Verification items for the finished model (mm, model axes). Give positions to 0.01 mm unless a question says otherwise; leave off trailing zeros. Loops run counter-clockwise (first coordinate to the right, second up) from the corner with the lowest first, then second, coordinate; pieces in that order, holes last. Notation, with made-up numbers: M 13,-14.5 L 49,-14.5 A23 ccw 49,-6.5 Z; hole C 43,44.25 d8. An arc over 180 degrees is marked long. Answer in a Markdown table with one row per item.
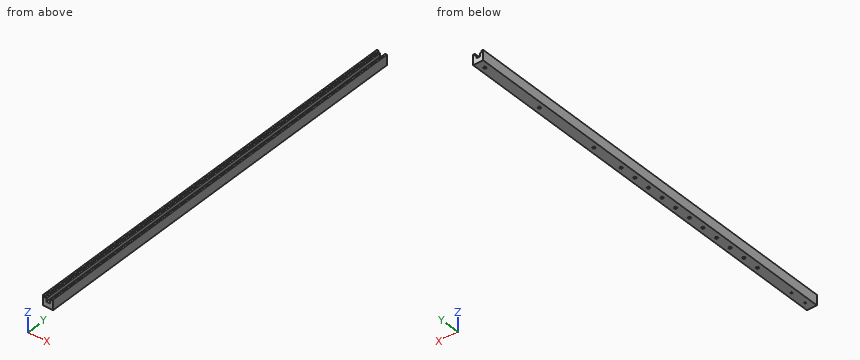
```python
from build123d import *

# Parameters (mm, degrees)
SKETCH1_W                 = 30
SKETCH1_H                 = 30
BOSS_EXTRUDE1_DEPTH       = 1225
CUT_EXTRUDE1_REACH        = 1227
SKETCH2_W                 = 20
SKETCH2_H                 = 5
CUT_EXTRUDE2_REACH        = 1227
SKETCH3_W                 = 10
SKETCH3_H                 = 10
SKETCH6_R                 = 4
CUT_EXTRUDE3_DEPTH        = 3
M6X1_0_TAPPED_HOLE1_D     = 5
M6X1_0_TAPPED_HOLE1_DEPTH = 15
M6X1_0_TAPPED_HOLE1_TIP   = 1.502151548


with BuildPart() as part:
    # Sketch1 → Boss-Extrude1 (new body)
    with BuildSketch(Plane(origin=(0, 0, 0), x_dir=(1, 0, 0), z_dir=(0, 1, 0))):
        Rectangle(SKETCH1_W, SKETCH1_H)
    extrude(amount=BOSS_EXTRUDE1_DEPTH)

    # Sketch2 → Cut-Extrude1 (cut, up to next)
    with BuildSketch(Plane(origin=(0, 1225, 0), x_dir=(1, 0, 0), z_dir=(0, 1, 0)), mode=Mode.PRIVATE) as cut_extrude1_sk1:
        with Locations((0, -12.5)):
            Rectangle(SKETCH2_W, SKETCH2_H)
    cut_extrude1_tool1 = extrude(cut_extrude1_sk1.sketch, amount=-CUT_EXTRUDE1_REACH, mode=Mode.PRIVATE) & part.part
    add(cut_extrude1_tool1.solids().sort_by_distance((0, 1225, 12.5))[0], mode=Mode.SUBTRACT)

    # Sketch3 → Cut-Extrude2 (cut, up to next)
    with BuildSketch(Plane(origin=(0, 1225, 0), x_dir=(1, 0, 0), z_dir=(0, 1, 0)), mode=Mode.PRIVATE) as cut_extrude2_sk1:
        with Locations((0, -5)):
            Rectangle(SKETCH3_W, SKETCH3_H)
    cut_extrude2_tool1 = extrude(cut_extrude2_sk1.sketch, amount=-CUT_EXTRUDE2_REACH, mode=Mode.PRIVATE) & part.part
    add(cut_extrude2_tool1.solids().sort_by_distance((0, 1225, 5))[0], mode=Mode.SUBTRACT)

    # Sketch6 → Cut-Extrude3 (cut)
    with BuildSketch(Plane(origin=(0, 0, -15), x_dir=(-1, 0, 0), z_dir=(0, 0, -1))):
        with Locations((0, 1200)):
            Circle(SKETCH6_R)
        with Locations((0, 1000)):
            Circle(SKETCH6_R)
        with Locations((0, 800)):
            Circle(SKETCH6_R)
        with Locations((0, 700)):
            Circle(SKETCH6_R)
        with Locations((0, 650)):
            Circle(SKETCH6_R)
        with Locations((0, 600)):
            Circle(SKETCH6_R)
        with Locations((0, 550)):
            Circle(SKETCH6_R)
        with Locations((0, 500)):
            Circle(SKETCH6_R)
        with Locations((0, 450)):
            Circle(SKETCH6_R)
        with Locations((0, 400)):
            Circle(SKETCH6_R)
        with Locations((0, 350)):
            Circle(SKETCH6_R)
        with Locations((0, 300)):
            Circle(SKETCH6_R)
        with Locations((0, 250)):
            Circle(SKETCH6_R)
        with Locations((0, 200)):
            Circle(SKETCH6_R)
    extrude(amount=-CUT_EXTRUDE3_DEPTH, mode=Mode.SUBTRACT)

    # M6x1.0 Tapped Hole1
    with Locations(Plane(origin=(0, 0, -15), x_dir=(-1, 0, 0), z_dir=(0, 0, -1))):
        with Locations((0, 75), (0, 25)):
            Hole(M6X1_0_TAPPED_HOLE1_D / 2, depth=M6X1_0_TAPPED_HOLE1_DEPTH)
            with Locations((0, 0, -(M6X1_0_TAPPED_HOLE1_DEPTH + M6X1_0_TAPPED_HOLE1_TIP / 2))):  # 118° drill point
                Cone(0, M6X1_0_TAPPED_HOLE1_D / 2, M6X1_0_TAPPED_HOLE1_TIP, mode=Mode.SUBTRACT)


solid = part.part
```
Item 1: Go/stop test with flat-tipped pins: pin 1 (8 mm diameter, centred on x = 2, y = 338, fed in from +Z); pin 2 (5 mm diameter, centred on x = 0, y = 250, fed in from +Z); pin 3 (6.5 mm diameter, centred on x = -0.5, y = 1201, fed in from -Z); pin 4 (6.5 mm diameter, centred on x = 0, y = 550, fed in from -Z). Record where each tip stops, or that it passes through.
Reported:
| item | result |
|---|---|
| pin 1 | stops at z = 10 |
| pin 2 | stops at z = 0 |
| pin 3 | stops at z = -15 |
| pin 4 | stops at z = -12 |
Item 2: Scan lines: L1, parallel to X at y = 1077.5, z = 7.25; L2, parallel to X at y = 800, z = -13.4; L3, parallel to Z at x = 2.5, y = 664. Record each from-to range of solid material in increasing order. Write a range as [from, to].
Reported:
| item | result |
|---|---|
| L1 | x = [-15, -5], [5, 15] |
| L2 | x = [-15, -4], [4, 15] |
| L3 | z = [-15, 0] |
Item 3: Sectioned sample at A-A (y = 953.5). Record the cut outline in (x, z).
Reported:
| item | result |
|---|---|
| outline | M -15,-15 L 15,-15 L 15,15 L 10,15 L 10,10 L 5,10 L 5,0 L -5,0 L -5,10 L -10,10 L -10,15 L -15,15 Z |
